```python
from build123d import *

# Parameters (mm, degrees)
EXTRUDE_START       = -4
EXTRUDE_1_DEPTH     = 8
SKETCH_2_R          = 5
CUT_EXTRUDE_1_DEPTH = 25.269322199


# Read off the part's stored shape, not the designer's step: 凸台-拉伸1
with BuildPart() as part:
    # 凸台-拉伸1 outline → 凸台-拉伸1 (new body)
    with BuildSketch(Plane.XY.offset(EXTRUDE_START)):
        Polygon((8.660254038, -15), (17.320508076, 0), (8.660254038, 15), (-8.660254038, 15), (-17.320508076, 0), (-8.660254038, -15), align=None)
    extrude(amount=EXTRUDE_1_DEPTH)

    # 草图2 → 切除-拉伸1 (cut, through all)
    with BuildSketch(Plane.XY.offset(4)):
        Circle(SKETCH_2_R)
    extrude(amount=-CUT_EXTRUDE_1_DEPTH, mode=Mode.SUBTRACT)


solid = part.part
```
Geometry check sheet. Reference: the model listing, model coordinates, mm. Coordinates: 2 decimals unless noted, no trailing zeros. Order: outer loops, then holes, each group sorted by start corner. A loop starts at its lowest first (then second) coordinate and runs counter-clockwise, first axis right, second up. Notation, with made-up numbers: (79, 85) - (106, 85) arc R11 cw to (106, 100) - close; hole circle Ø1 at (61.5, 24.5). An arc over 180 degrees is marked (long way). Answer in a Markdown table with one row per item. Add a question column.
1. Gauge pin test, flat ends, axial feed: pin 1 Ø1 at (y, z) = (-1.5, -3) entering from +X; pin 2 Ø9 at (x, y) = (0, 0) entering from +Z. Record the tip position at first contact, or that the pin passes through.
2. Section check D-D (y = -12.5). Enter the section's corners in (x, z), plus the area to 3 significant figures.
3. Section check C-C (y = 4.5). Enter the section's corners in (x, z), plus the area to 3 significant figures.
4. Material ranges on L1, parallel to Y at x = 0, z = 1.75; L2, parallel to Y at x = -1.5, z = -1; L3, parallel to X at y = 0.25, z = -2, recorded low to high. Write a range as [from, to].
5. Section check B-B (z = 1). Enter the section's corners in (x, y), plus the area to 3 significant figures.
6. Section check A-A (x = 0). Enter the section's corners in (y, z), plus the area to 3 significant figures.
7. Draft check along Y on faces 1 (the face through (-13.05, -7.4, -0.06)), 2 (the face through (-1.08, -4.88, 0.06)), 3 (the face through (4, 4, -4)). Enter one of: +Y half, -Y half, draft (parallel to the pull), parting line (faces both ways), or undercut.
Data:
| question | item | result |
|---|---|---|
| 1 | pin 1 | stops at x = 16.74 |
| 1 | pin 2 | passes through |
| 2 | outline | (-10.1, -4) - (10.1, -4) - (10.1, 4) - (-10.1, 4) - close |
| 2 | area | 162 mm² |
| 3 | outline | (-14.72, -4) - (-2.18, -4) - (-2.18, 4) - (-14.72, 4) - close; (2.18, -4) - (14.72, -4) - (14.72, 4) - (2.18, 4) - close |
| 3 | area | 201 mm² |
| 4 | L1 | y = [-15, -5], [5, 15] |
| 4 | L2 | y = [-15, -4.77], [4.77, 15] |
| 4 | L3 | x = [-17.18, -4.99], [4.99, 17.18] |
| 5 | outline | (-17.32, 0) - (-8.66, -15) - (8.66, -15) - (17.32, 0) - (8.66, 15) - (-8.66, 15) - close; hole circle Ø10 at (0, 0) |
| 5 | area | 701 mm² |
| 6 | outline | (-15, -4) - (-5, -4) - (-5, 4) - (-15, 4) - close; (5, -4) - (15, -4) - (15, 4) - (5, 4) - close |
| 6 | area | 160 mm² |
| 7 | face 1 | -Y half |
| 7 | face 2 | undercut |
| 7 | face 3 | draft |
